Verification items for the finished model (mm, model axes). Face numbers are marked on the shaded views. A direction names the side the tool comes from. Coordinates: 2 decimals unless noted, no trailing zeros. Loops run counter-clockwise (first coordinate to the right, second up) from the corner with the lowest first, then second, coordinate; pieces in that order, holes last. Notation, with made-up numbers: (44.5, 57) -> (65.5, 57) arc R21 cw to (65.5, 86) -> close; hole circle Ø8 at (32.25, 34.5). An arc over 180 degrees is marked (long way). Write item = value, one per line.
```python
from build123d import *

# Parameters (mm, degrees)
F1_DEPTH     = 406.4
F2_T1_DEPTH  = 417.5993599931
F2_T3_DEPTH  = 355.6
F2_T5_DEPTH  = 163.5993599931
F2_T7_DEPTH  = 533.4
F2_T12_DEPTH = 25.4
F2_T18_DEPTH = 25.4
F3_W         = 89.2188286402
F3_H         = 154.1103798959
F4_DEPTH     = 127


# Not quite as in the source:
# - a fillet or chamfer that OpenCascade refuses, or shapes differently, is made with other operations: its cross-section is extruded or revolved along the edge and cut away or added
# - a feature names something its author has since deleted; it is built from what else it names


with BuildPart() as f1:
    # F0 (on Right) → F1 (new body)
    with BuildSketch(Plane.YZ):
        Polygon((113.1009757519, -66.1072761975), (126.957971921, 39.0469668974), (-253.4152170727, 60.8927238025), (-253.4152170727, -66.1072761975), align=None)
    extrude(amount=F1_DEPTH)

    # F2: fillet of radius 25.4 on 6 edges, made by hand

    # F2_s2 → F2_t1 (cut)
    with BuildSketch(Plane(origin=(0, 187.7009218342, -10.780120229), x_dir=(1, 0, 0), z_dir=(0, -0.9983548268, 0.0573379446))):
        with BuildLine():
            ThreePointArc((25.4, 46.2622370369), (7.4394877579, 38.822749279), (0, 20.8622370369))
            Line((0, 20.8622370369), (0, 46.2622370369))
            Line((0, 46.2622370369), (25.4, 46.2622370369))
        make_face()
        with BuildLine():
            ThreePointArc((381, 46.2622370369), (398.9605122421, 38.822749279), (406.4, 20.8622370369))
            Line((406.4, 20.8622370369), (406.4, 46.2622370369))
            Line((406.4, 46.2622370369), (381, 46.2622370369))
        make_face()
    extrude(amount=F2_T1_DEPTH, mode=Mode.SUBTRACT)

    # F2_s4 → F2_t3 (cut)
    with BuildSketch(Plane.YZ.offset(25.4)):
        with BuildLine():
            ThreePointArc((-226.558833279, 59.3502963952), (-245.4532194187, 52.4603288172), (-253.4152170727, 33.9920837956))
            Line((-253.4152170727, 33.9920837956), (-253.4152170727, 60.8927238025))
            Line((-253.4152170727, 60.8927238025), (-226.558833279, 59.3502963952))
        make_face()
    extrude(amount=F2_T3_DEPTH, mode=Mode.SUBTRACT)

    # F2_s6 → F2_t5 (cut)
    with BuildSketch(Plane.XY.offset(-129.6072761975)):
        with BuildLine():
            ThreePointArc((25.4, -253.4152170727), (7.4394877579, -245.9757293148), (0, -228.0152170727))
            Line((0, -228.0152170727), (0, -253.4152170727))
            Line((0, -253.4152170727), (25.4, -253.4152170727))
        make_face()
        with BuildLine():
            ThreePointArc((381, -253.4152170727), (398.9605122421, -245.9757293148), (406.4, -228.0152170727))
            Line((406.4, -228.0152170727), (406.4, -253.4152170727))
            Line((406.4, -253.4152170727), (381, -253.4152170727))
        make_face()
    extrude(amount=F2_T5_DEPTH, mode=Mode.SUBTRACT)

    # F2_s8 → F2_t7 (cut)
    with BuildSketch(Plane.YZ.offset(-63.5)):
        with BuildLine():
            ThreePointArc((-253.4152170727, -40.7072761975), (-245.9757293148, -58.6677884397), (-228.0152170727, -66.1072761975))
            Line((-228.0152170727, -66.1072761975), (-253.4152170727, -66.1072761975))
            Line((-253.4152170727, -66.1072761975), (-253.4152170727, -40.7072761975))
        make_face()
    extrude(amount=F2_T7_DEPTH, mode=Mode.SUBTRACT)


with BuildPart() as f2_tool10:
    # F2_s11 → F2_t12 (new body)
    with BuildSketch(Plane.YZ.offset(25.4)):
        Polygon((-228.0152170727, 33.9920837956), (-226.558833279, 59.3502963952), (-253.4152170727, 60.8927238025), (-253.4152170727, 33.9920837956), align=None)
    extrude(amount=-F2_T12_DEPTH)

    # F2_s13 → F2_t14 (revolve, cut)
    with BuildSketch(Plane(origin=(25.4, -228.0152170727, 33.9920837956), x_dir=(0, 0.6865355254, -0.7270962607), z_dir=(0, 0.7270962607, 0.6865355254))):
        with BuildLine():
            ThreePointArc((0, -25.4), (25.4, 0), (0, 25.4))
            Line((0, 25.4), (0, -25.4))
        make_face()
    revolve(axis=Axis((25.4, -228.0152170727, 33.9920837956), (-1, 0, 0)), mode=Mode.SUBTRACT)


with BuildPart() as f1_1:
    add(f1.part)

    # F2_t9: cut F2_tool10
    add(f2_tool10.part, mode=Mode.SUBTRACT)


with BuildPart() as f2_tool16:
    # F2_s17 → F2_t18 (new body)
    with BuildSketch(Plane.YZ.offset(381)):
        Polygon((-228.0152170727, 33.9920837956), (-226.558833279, 59.3502963952), (-253.4152170727, 60.8927238025), (-253.4152170727, 33.9920837956), align=None)
    extrude(amount=F2_T18_DEPTH)

    # F2_s19 → F2_t20 (revolve, cut)
    with BuildSketch(Plane(origin=(381, -228.0152170727, 33.9920837956), x_dir=(0, 0.6865355254, -0.7270962607), z_dir=(0, -0.7270962607, -0.6865355254))):
        with BuildLine():
            ThreePointArc((0, -25.4), (25.4, 0), (0, 25.4))
            Line((0, 25.4), (0, -25.4))
        make_face()
    revolve(axis=Axis((381, -228.0152170727, 33.9920837956), (1, 0, 0)), mode=Mode.SUBTRACT)


with BuildPart() as f1_2:
    add(f1_1.part)

    # F2_t15: cut F2_tool16
    add(f2_tool16.part, mode=Mode.SUBTRACT)

    # F3 (on face) → F4 (cut)
    with BuildSketch(Plane(origin=(0, 0, -66.1072761975), x_dir=(1, 0, 0), z_dir=(0, 0, -1))):
        with Locations((-6.5094143201, -113.9561656998)):
            Rectangle(F3_W, F3_H)
        with Locations((412.9094143201, -113.9561656998)):
            Rectangle(F3_W, F3_H)
    extrude(amount=-F4_DEPTH, mode=Mode.SUBTRACT)


solid = f1_2.part
```
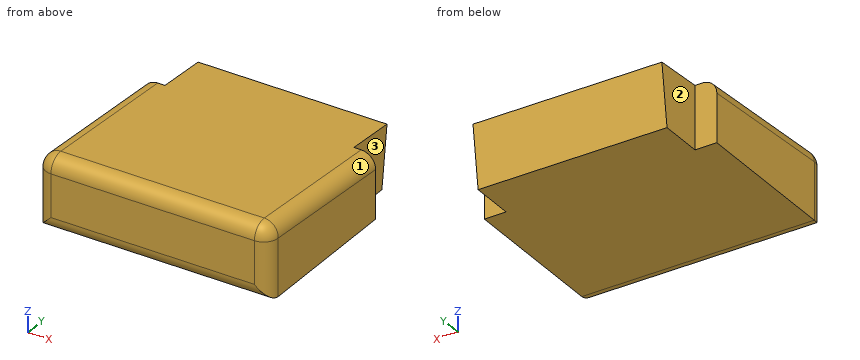
1) Sectioned sample at D-D, the plane x = 244. Record the cut outline in (y, z), plus the area to 3 significant figures.
Ans:
outline = (-253.42, -40.71) arc R25.4 ccw to (-228.02, -66.11) -> (113.1, -66.11) -> (126.96, 39.05) -> (-226.56, 59.35) arc R25.4 ccw to (-253.42, 33.99) -> close
area = 43,100 mm2
2) Sectioned sample at A-A, the plane x = 32. Record the cut outline in (y, z), plus the area to 3 significant figures.
Ans:
outline = (-253.42, -40.71) arc R25.4 ccw to (-228.02, -66.11) -> (36.9, -66.11) -> (36.9, 44.22) -> (-226.56, 59.35) arc R25.4 ccw to (-253.42, 33.99) -> close
area = 34,200 mm2
3) Sectioned sample at C-C, the plane z = -27. Record the cut outline in (x, y).
Ans:
outline = (0, -228.02) arc R25.4 ccw to (25.4, -253.42) -> (381, -253.42) arc R25.4 ccw to (406.4, -228.02) -> (406.4, 36.9) -> (368.3, 36.9) -> (368.3, 118.25) -> (38.1, 118.25) -> (38.1, 36.9) -> (0, 36.9) -> close
4) Sectioned sample at B-B, the plane z = -47. Record the cut outline in (x, y), plus the area to 3 significant figures.
Ans:
outline = (0, -228.02) arc R25.4 ccw to (19.11, -252.62) -> (387.29, -252.62) arc R25.4 ccw to (406.4, -228.02) -> (406.4, 36.9) -> (368.3, 36.9) -> (368.3, 115.62) -> (38.1, 115.62) -> (38.1, 36.9) -> (0, 36.9) -> close
area = 143,000 mm2
5) Material ranges on line 1 (X direction, y = 46, z = 22); line 2 (Z direction, x = 211, y = -222); line 3 (Y direction, x = 99.5, z = -46.5), recorded low to high.
Ans:
line_1 = 38.1 to 368.3
line_2 = -66.11 to 59.09
line_3 = -252.75 to 115.68
6) Depth check by flat-ended pin: pin 1 Ø1 at (x, y) = (289, -150) entering from +Z; pin 2 Ø19 at (x, z) = (389, -17) entering from +Y; pin 3 Ø2 at (x, z) = (94, -19.5) entering from +Y; pin 4 Ø10 at (x, z) = (312.5, 35.5) entering from -Y. Enter the tip coordinate at first touch or a pass-through.
Ans:
pin_1 = 54.98
pin_2 = 36.9
pin_3 = 119.37
pin_4 = -253.42
7) Tool access check on the marked faces 1, 2 and 3. Record the directions out of +Z, -Z, +X, -X, +Y, -Y that give a thin tool (end or side, any length) a straight path to the whole face; none if there is none.
Ans:
face_1 = +Z, +X, +Y
face_2 = +Z, -Z, -X, +Y
face_3 = +Z, -Z, +X, +Y
